Check sheet for the modelled part. Datum: model origin and axes. Units: mm. Round coordinates to 2 decimals unless told otherwise and drop trailing zeros. Write each loop counter-clockwise with the first axis right and the second up, starting at its lowest first coordinate (ties: lowest second). Pieces come first, ordered by that corner, then holes. Notation, with made-up numbers: (-39, -24) -> (5, -24) arc R25 cw to (5, -11) -> close; hole circle Ø2 at (82.25, 49). An arc over 180 degrees is marked (long way). One line per item, written item: value.
from build123d import *

# Parameters (mm, degrees)
PAD_DEPTH = 11.75
FILLET_R  = 2


with BuildPart() as part:
    # Sketch (on XZ_Plane of Origin) → Pad (new body)
    with BuildSketch(Plane.XZ):
        Polygon((-32.25, 5.875), (-32.25, -5.875), (32.25, -5.875), (32.25, -2.375), (16.25, 5.875), align=None)
    extrude(amount=PAD_DEPTH)

    # Fillet
    fillet_edges = [part.edges().sort_by_distance(p)[0] for p in [
        (32.25, 0, -4.125),
        (32.25, -11.75, -4.125),
        (32.25, -5.875, -2.375),
        (24.25, -11.75, 1.75),
        (24.25, 0, 1.75),
        (16.25, -5.875, 5.875),
        (-8, -11.75, 5.875),
        (-8, 0, 5.875),
        (-32.25, 0, 0),
        (-32.25, -5.875, 5.875),
        (-32.25, -11.75, 0),
    ]]
    fillet(fillet_edges, radius=FILLET_R)


solid = part.part
Item 1: Depth check by flat-ended pin: P1, Ø1.5, axis at x = -18.5, y = -10, coming from the +Z side (3 decimals). Enter the tip coordinate at first touch or a pass-through.
Answer:
P1: stops at z = 5.875
Item 2: Sectioned sample at A-A on y = -6.5. Enter the section's corners in (x, z) (3 decimals).
Answer:
outline: (-32.25, -5.875) -> (32.25, -5.875) -> (32.25, -3.594) arc R2 ccw to (31.167, -1.816) -> (16.681, 5.653) arc R2 ccw to (15.765, 5.875) -> (-30.25, 5.875) arc R2 ccw to (-32.25, 3.875) -> close
Item 3: Thickness scan on line 1 (Z direction, x = -10.5, y = -10.75) (3 decimals); line 2 (Y direction, x = 21, z = 1.5); line 3 (Z direction, x = -13.5, y = -10.5) (3 decimals). Record the ranges inside material, lowest first.
Answer:
line 1: z = -5.875 to 5.607
line 2: y = -11.73 to -0.02
line 3: z = -5.875 to 5.729
Item 4: Sectioned sample at B-B on y = -10.5. Enter the section's corners in (x, z) (3 decimals), and give its area (3 significant figures).
Answer:
outline: (-32.104, -5.875) -> (32.104, -5.875) -> (32.104, -3.594) arc R1.854 ccw to (31.1, -1.946) -> (16.614, 5.523) arc R1.854 ccw to (15.765, 5.729) -> (-30.25, 5.729) arc R1.854 ccw to (-32.104, 3.875) -> close
area: 679 mm^2
